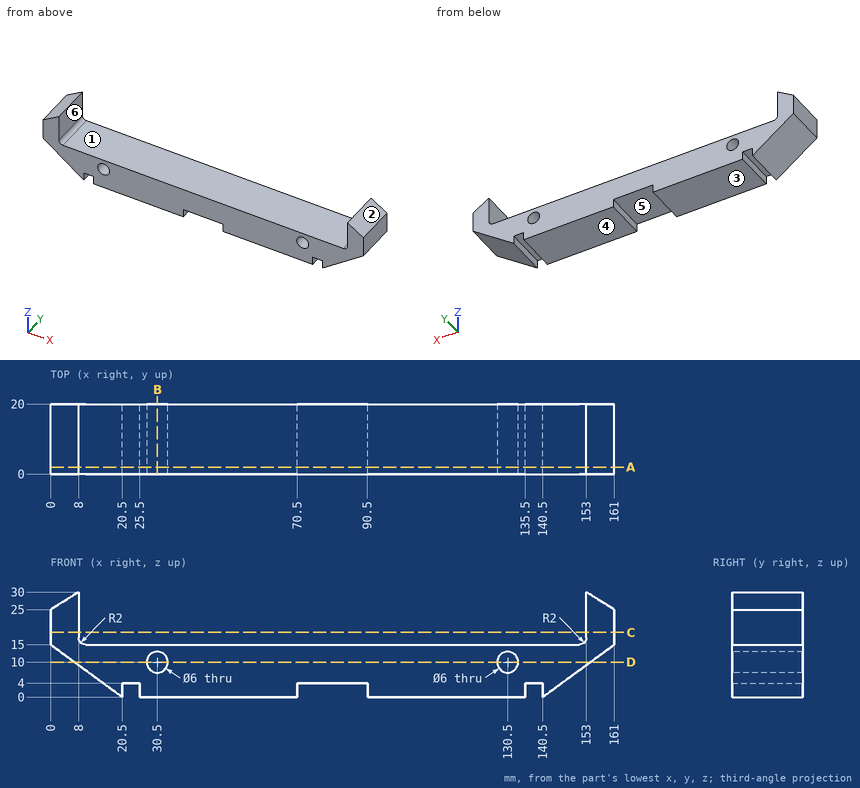
The figure shows three views and two pictorial views of one solid part (mm, origin at its lowest corner). Answer the questions. A direction names the side the tool comes from. Coordinates: 2 decimals unless noted, no trailing zeros. Order: outer loops, then holes, each group sorted by start corner. A loop starts at its lowest first (then second) coordinate and runs counter-clockwise, first axis right, second up.
Q1. A cutting plane is placed at A-A, the plane y = 2. Write down the section's boundary in (x, z).
Q2. A cutting plane is placed at C-C, the plane z = 18.5. Write down the section's boundary in (x, y).
Q3. For a pull along X with two mould halves and no side action, classify the marked faces 1, 2 and 3 as pulls with the +X half, pulls with the -X half, needs draft (parallel to the pull), parting line crosses it, or undercut.
Q4. Consider line 1 (Z direction, x = 130.5, y = 11); line 2 (X direction, y = 17.75, z = 24.5); line 3 (X direction, y = 13.25, z = 7.5). Determine where each line is inside the solid, lowest interval first.
Q5. Given P1, Ø5, axis at y = 3, z = 6, coming from the +X side; P2, Ø6, axis at x = 140.5, y = 11.5, coming from the +Z side; P3, Ø4.5, axis at y = 6, z = 2.5, coming from the +X side; P4, Ø3.5, axis at x = 30.5, z = 10, coming from the -Y side, each flat-ended and moving along its own axis, determine where each tip first touches the part or whether it passes through.
Q6. A cutting plane is placed at B-B, the plane x = 30.5. Write down the section's boundary in (y, z), and give its area (3 significant figures).
Q7. A cutting plane is placed at D-D, the plane z = 10. Write down the section's boundary in (x, y), and give its area (3 significant figures).
Q8. Which of the six approach directions +Z, -Z, +X, -X, +Y, -Y give full straight-line access (tool end or side, diameter ignored) to the marked faces 4, 5 and 6?
Answers follow:
1. outline: (0, 15) - (20.5, 0) - (20.5, 4) - (25.5, 4) - (25.5, 0) - (70.5, 0) - (70.5, 4) - (90.5, 4) - (90.5, 0) - (135.5, 0) - (135.5, 4) - (140.5, 4) - (140.5, 0) - (161, 15) - (161, 25) - (153, 30) - (153, 17) arc R2 cw to (151, 15) - (10, 15) arc R2 cw to (8, 17) - (8, 30) - (0, 25) - close; hole circle Ø6 at (30.5, 10); hole circle Ø6 at (130.5, 10)
2. outline: (0, 0) - (8, 0) - (8, 20) - (0, 20) - close; (153, 0) - (161, 0) - (161, 20) - (153, 20) - close
3. face 1: undercut
3. face 2: pulls with the +X half
3. face 3: needs draft
4. line 1: z = 0 to 7, 13 to 15
4. line 2: x = 0 to 8, 153 to 161
4. line 3: x = 10.25 to 28.84, 32.16 to 128.84, 132.16 to 150.75
5. P1: stops at x = 152.12
5. P2: stops at z = 15
5. P3: stops at x = 146.99
5. P4: passes through
6. outline: (0, 0) - (20, 0) - (20, 7) - (0, 7) - close; (0, 13) - (20, 13) - (20, 15) - (0, 15) - close
6. area: 180 mm2
7. outline: (6.83, 0) - (27.5, 0) - (27.5, 20) - (6.83, 20) - close; (33.5, 0) - (127.5, 0) - (127.5, 20) - (33.5, 20) - close; (133.5, 0) - (154.17, 0) - (154.17, 20) - (133.5, 20) - close
7. area: 2,710 mm2
8. face 4: -Z, +X, -X, +Y, -Y
8. face 5: -Z, +Y, -Y
8. face 6: +Z, +Y, -Y
